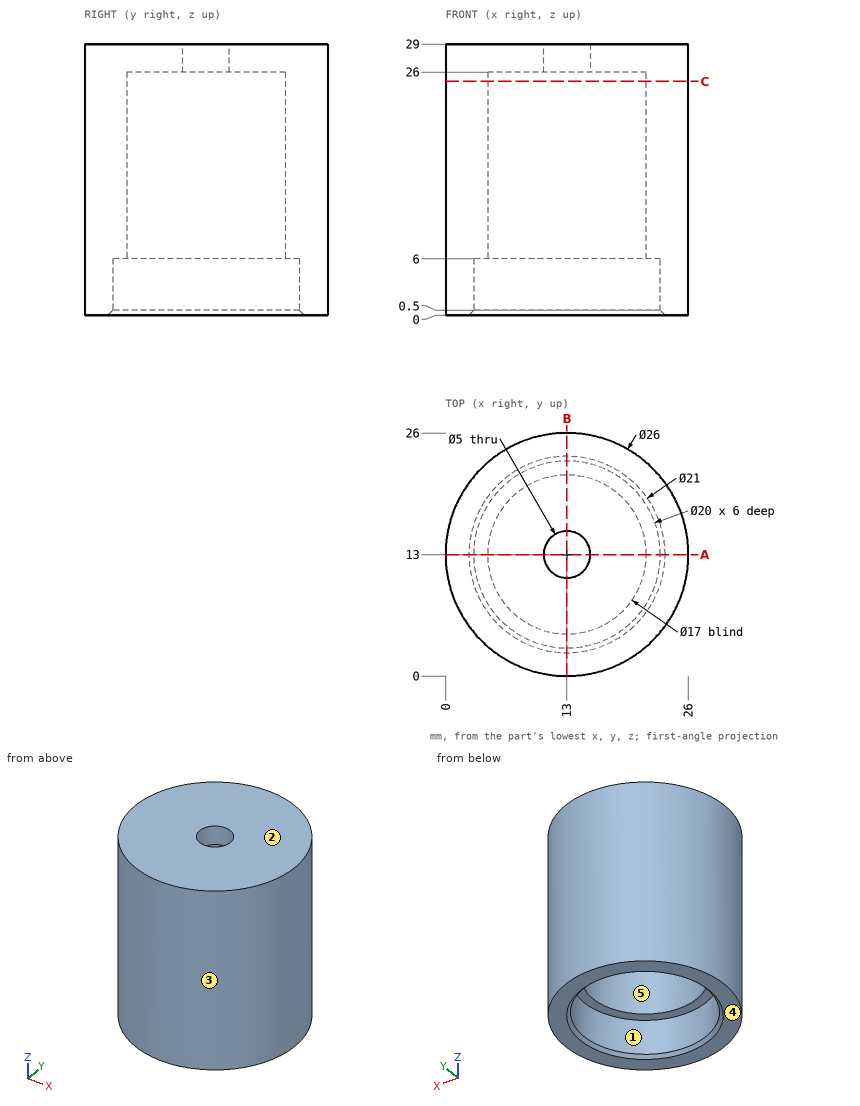
Design review of the part shown in the three views and the two pictorial views. Dimensions are in mm from the part's minimum x, y and z. A direction names the side the tool comes from. Round coordinates to 2 decimals unless told otherwise and drop trailing zeros. Order: outer loops, then holes, each group sorted by start corner. A loop starts at its lowest first (then second) coordinate and runs counter-clockwise, first axis right, second up.
Q1. Wall thickness on line 1 (Y direction, x = 13, z = 12.75); line 2 (Y direction, x = 13, z = 27.9); line 3 (Z direction, x = 14.5, y = 4.25): over which ranges is each line inside the solid? List them lowest first.
Findings below:
line 1: y = 0 to 4.5, 21.5 to 26
line 2: y = 0 to 10.5, 15.5 to 26
line 3: z = 6 to 29
Q2. We need section C-C, the plane z = 25. Give the boundary of the cut face in (x, y), plus the area to 3 significant figures.
Findings below:
outline: circle Ø26 at (13, 13); hole circle Ø17 at (13, 13)
area: 304 mm2
Q3. Mouldability with a two-part tool opening along Y and no side actions: class the marked faces 1, 2 and 3 as pulls with the +Y half, pulls with the -Y half, needs draft (parallel to the pull), parting line crosses it, or undercut.
Findings below:
face 1: undercut
face 2: needs draft
face 3: parting line crosses it
Q4. Machinability: for the marked faces 4 and 5, which of the approach directions +Z, -Z, +X, -X, +Y, -Y give a long, thin tool a straight path to every point of the face, cutting with its end or side? Answer none if there is none.
Findings below:
face 4: -Z, +X, -X, +Y, -Y
face 5: -Z
Q5. We need section A-A, the plane y = 13. Give the boundary of the cut face in (x, z), plus the area to 3 significant figures.
Findings below:
outline: (0, 0) - (2.5, 0) - (3, 0.5) - (3, 6) - (4.5, 6) - (4.5, 26) - (10.5, 26) - (10.5, 29) - (0, 29) - close; (15.5, 26) - (21.5, 26) - (21.5, 6) - (23, 6) - (23, 0.5) - (23.5, 0) - (26, 0) - (26, 29) - (15.5, 29) - close
area: 279 mm2
Q6. Insertion check: P1, Ø1.5, axis at y = 8.5, z = 22.5, coming from the -X side; P2, Ø4, axis at y = 8, z = 11, coming from the +X side; P3, Ø6, axis at x = 9.5, z = 24, coming from the +Y side; P4, Ø1, axis at x = 5, y = 22.5, coming from the -Z side. Each pin has a flat end and moves straight along its axis. Give the tip position at first contact, or say it passes through.
Findings below:
P1: stops at x = 0.55
P2: stops at x = 25.65
P3: stops at y = 25.99
P4: stops at z = 0
